from build123d import *

# Parameters (mm, degrees)
SKETCH107_R             = 9.5
SKETCH107_R_2           = 11
SKETCH107_R_3           = 1.65
SKETCH107_R_4           = 1.6
PAD033_DEPTH            = 120
POCKET065_DEPTH         = 152.4
SKETCH104_R             = 3.1
SKETCH104_R_2           = 14
POCKET063_DEPTH         = 8
SKETCH103_R             = 11.15
POCKET064_DEPTH         = 5
SKETCH106_R             = 11.15
POCKET066_DEPTH         = 5
CHAMFER013_SIZE         = 0.8
BODY025_PLACEMENT_ANGLE = 90


with BuildPart() as part:
    # Sketch107 → Pad033 (new body)
    with BuildSketch(Plane.XY):
        with BuildLine():
            Line((-50, 0), (50, 0))
            Line((50, 0), (30, 215))
            ThreePointArc((30, 215), (0, 241.8364621975), (-30, 215))
            Line((-50, 0), (-30, 215))
        make_face()
        with Locations((0, 221.15)):
            Circle(SKETCH107_R, mode=Mode.SUBTRACT)
        with Locations((0, 21.15)):
            Circle(SKETCH107_R_2, mode=Mode.SUBTRACT)
        with Locations((0, 101.15)):
            Circle(SKETCH107_R, mode=Mode.SUBTRACT)
        with Locations((-15.5, 36.65)):
            Circle(SKETCH107_R_3, mode=Mode.SUBTRACT)
        with Locations((15.5, 36.65)):
            Circle(SKETCH107_R_3, mode=Mode.SUBTRACT)
        with Locations((-30.5906976744, 101.15)):
            Circle(SKETCH107_R_4, mode=Mode.SUBTRACT)
        with Locations((30.5906976744, 101.15)):
            Circle(SKETCH107_R_4, mode=Mode.SUBTRACT)
        with Locations((-25.0093023256, 161.15)):
            Circle(SKETCH107_R_4, mode=Mode.SUBTRACT)
        with Locations((25.0093023256, 161.15)):
            Circle(SKETCH107_R_4, mode=Mode.SUBTRACT)
    extrude(amount=PAD033_DEPTH)

    # Sketch105 → Pocket065 (cut, symmetric)
    with BuildSketch(Plane(origin=(0, 0, 120), x_dir=(0, 0, -1), z_dir=(1, 0, 0))):
        Polygon((7, 252.37), (113, 252.37), (113, 9), (111, 7), (9, 7), (7, 9), align=None)
    extrude(amount=POCKET065_DEPTH, both=True, mode=Mode.SUBTRACT)

    # Sketch104 (on Face1 of Pocket065) → Pocket063 (cut)
    with BuildSketch(Plane.XZ):
        with Locations((-40, 100)):
            Circle(SKETCH104_R)
        with Locations((40, 100)):
            Circle(SKETCH104_R)
        with Locations((-40, 20)):
            Circle(SKETCH104_R)
        with Locations((40, 20)):
            Circle(SKETCH104_R)
        with Locations((0, 60)):
            Circle(SKETCH104_R_2)
    extrude(amount=-POCKET063_DEPTH, mode=Mode.SUBTRACT)

    # Sketch103 (on Face4 of Pocket063) → Pocket064 (cut)
    with BuildSketch(Plane.XY.offset(120)):
        with Locations((0, 101.15)):
            Circle(SKETCH103_R)
        with Locations((0, 221.15)):
            Circle(SKETCH103_R)
    extrude(amount=-POCKET064_DEPTH, mode=Mode.SUBTRACT)

    # Sketch106 (on Face3 of Pocket064) → Pocket066 (cut)
    with BuildSketch(Plane(origin=(0, 0, 0), x_dir=(1, 0, 0), z_dir=(0, 0, -1))):
        with Locations((0, -221.15)):
            Circle(SKETCH106_R)
        with Locations((0, -101.15)):
            Circle(SKETCH106_R)
    extrude(amount=-POCKET066_DEPTH, mode=Mode.SUBTRACT)

    # Chamfer013
    chamfer013_edges = [part.edges().sort_by_distance(p)[0] for p in [
        (23.409302, 161.15, 0),
        (28.990698, 101.15, 0),
        (23.409302, 161.15, 120),
        (28.990698, 101.15, 120),
    ]]
    chamfer(chamfer013_edges, length=CHAMFER013_SIZE)


with BuildPart() as part_1:
    # Body025 placement: moved
    add(part.part.moved(Location((1, 0, 0))).rotate(Axis((1, 0, 0), (1, 0, 0)), BODY025_PLACEMENT_ANGLE))


solid = part_1.part
The model under review builds one solid part; all positions refer to its coordinate system, in mm. A direction names the side the tool comes from. Round coordinates to 2 decimals unless told otherwise and drop trailing zeros. Order: outer loops, then holes, each group sorted by start corner. A loop starts at its lowest first (then second) coordinate and runs counter-clockwise, first axis right, second up. Notation, with made-up numbers: (-31, 39) - (0, 39) arc R35 ccw to (0, 75) - close; hole circle Ø9 at (8, 39). An arc over 180 degrees is marked (long way). Use one line per item in the form item = value.
Q1. Add section A-A on y = -100. Give the boundary of the cut face in (x, z).
Response values:
outline = (-49, 0) - (-42.1, 0) - (-42.1, 7) - (-48.35, 7) - close; (-35.9, 0) - (37.9, 0) - (37.9, 7) - (-35.9, 7) - close; (44.1, 0) - (51, 0) - (50.35, 7) - (44.1, 7) - close
Q2. Add section B-B on z = 21.15. Give the boundary of the cut face in (x, y), then the cut area to 3 significant figures.
Response values:
outline = (-47.03, -120) - (-10, -120) - (-10, -113) - (-47.03, -113) - close; (-47.03, -7) - (-10, -7) - (-10, 0) - (-47.03, 0) - close; (12, -120) - (49.03, -120) - (49.03, -113) - (12, -113) - close; (12, -7) - (49.03, -7) - (49.03, 0) - (12, 0) - close
area = 1,040 mm^2
Q3. Tool access review of faces 1 (the flat face through (2, -113, 124)), 2 (the cylindrical face through (6.914, -3.451, 30.425)), 3 (the flat face through (-4, -5, 92.8)), 4 (the flat face through (10, -115, 105)): name each direction out of +Z, -Z, +X, -X, +Y, -Y from which nothing blocks a thin tool from reaching the whole face with its end or side.
Response values:
face_1 = +Z, +X, -X
face_2 = +Y, -Y
face_3 = +Y
face_4 = -Y
Q4. Mouldability with a two-part tool opening along Y and no side actions: class faces 5 (the flat face through (0, -120, 123)), 6 (the cylindrical face through (6.994, -2.465, 211.748)), 7 (the cylindrical face through (-2.03, -46.33, 3.45)) as pulls with the +Y half, pulls with the -Y half, needs draft (parallel to the pull), parting line crosses it, or undercut.
Response values:
face_5 = pulls with the -Y half
face_6 = needs draft
face_7 = undercut
Q5. Add section D-D on y = -52.5. Give the boundary of the cut face in (x, z), then the cut area to 3 significant figures.
Response values:
outline = (-49, 0) - (-10.82, 0) - (-10.82, 7) - (-48.35, 7) - close; (12.82, 0) - (51, 0) - (50.35, 7) - (12.82, 7) - close
area = 530 mm^2
Q6. Add section C-C on x = 1. Give the number of separate pieces and of enclosed holes in the cut face, then the cut area to 3 significant figures.
Response values:
separate_pieces = 8
enclosed_holes = 0
area = 3,030 mm^2
Q7. Clearance check with a flat-ended pin moving along its axis: P1, Ø5, axis at x = -25.5, y = -44.5, coming from the +Z side. State where the tip first meets the part, or that it passes through.
Response values:
P1 = 7
Q8. To check wall thickness, follow line 1 (Y direction, x = -12, z = 180); line 2 (Z direction, x = 6, y = -114); line 3 (X direction, y = -2.25, z = 161.15). State the ranges of each line that lie inside material, in increasing order.
Response values:
line_1 = -120 to -113, -7 to 0
line_2 = 0 to 11.35, 30.95 to 93.07, 109.23 to 213.07, 229.23 to 241.42
line_3 = -34.01 to -25.61, -22.41 to 24.41, 27.61 to 36.01
